Could you check a few things on this drawing? It's one solid part, dimensions in mm from its lowest x, y, z. A direction names the side the tool comes from. Coordinates: 2 decimals unless noted, no trailing zeros. Write each loop counter-clockwise with the first axis right and the second up, starting at its lowest first coordinate (ties: lowest second). Pieces come first, ordered by that corner, then holes. Notation, with made-up numbers: (44, 75) - (56, 75) arc R18 ccw to (56, 108) - close; hole circle Ø1 at (37.25, 79.25). An arc over 180 degrees is marked (long way). Answer as a JSON object with one key per item and string values. Group by question number.
1) If we section it at B-B (z = 8.75): Write out the boundary of the cut face in (x, y).
2) Please list where these lines run through material, in increasing order: line 1 along Z through (x, y) = (6, 2); line 2 along Z through (x, y) = (1.5, 30) (3 decimals); line 3 along Z through (x, y) = (2.5, 5.5) (3 decimals).
3) If we section it at A-A (x = 5.25): Write out the boundary of the cut face in (y, z) (3 decimals).
4) On a 3-axis mill with a long thin cutter (end or side, diameter ignored), from which of +Z, -Z, +X, -X, +Y, -Y can I reach the whole of each face in a straight line? I mean the marked faces 5 and 6. Say none if no direction works.
5) We'd pull the mould along Z, two halves only. Please class the marked faces 1, 2, 3 and 4: released by +Z, released by -Z, zero draft, split by the parting line, or undercut.
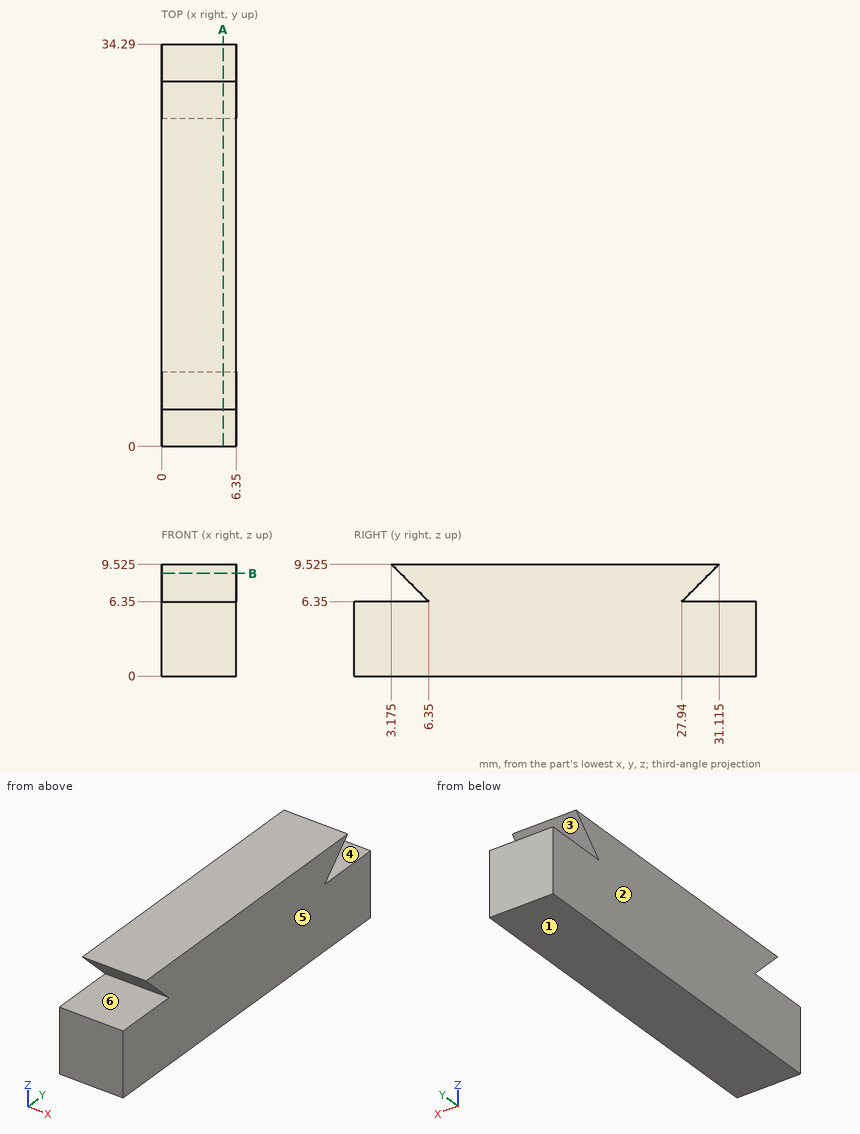
Here are the results:
{
 "1": {"outline": "(0, 3.95) - (6.35, 3.95) - (6.35, 30.34) - (0, 30.34) - close"},
 "2": {"line 1": "z = 0 to 6.35", "line 2": "z = 0 to 6.35, 8.41 to 9.525", "line 3": "z = 0 to 6.35, 7.2 to 9.525"},
 "3": {"outline": "(0, 0) - (34.29, 0) - (34.29, 6.35) - (27.94, 6.35) - (31.115, 9.525) - (3.175, 9.525) - (6.35, 6.35) - (0, 6.35) - close"},
 "4": {"face 5": "+Z, -Z, +X, +Y, -Y", "face 6": "+X, -X, -Y"},
 "5": {"face 1": "released by -Z", "face 2": "zero draft", "face 3": "undercut", "face 4": "undercut"}
}
